Solid Edge part; units mm, degrees
sketch "Sketch1" plane through (0, 0, 0) normal (0, 0, 1) x (1, 0, 0)
  line L0 (-16, -30) -> (16, -30)
  line L1 (16, -30) -> (16, 30)
  line L2 (16, 30) -> (-16, 30)
  line L3 (-16, 30) -> (-16, -30)
  dimension "D1" = 16
  dimension "D2" = 16
extrude "Protrusion1" add sketch "Sketch1" along normal blind 73
sketch "Sketch2" plane through (0, 0, 73) normal (0, 0, 1) x (1, 0, 0)
  circle A0 centre (0, -20) radius 2.35
  circle A1 centre (0, -2) radius 2.35
extrude "Extrusionsausschnitt_1" cut sketch "Sketch2" against normal blind 36
chamfer "Fase_3" distance 0.7 angle 60 2 edges at (-2.35, -2, 73) (-2.35, -20, 73) measured on face at (-10.9867, -19.4, 73)
chamfer "Fase_6" distance 3 angle 45 4 edges at (-16, 0, 73) (-16, 0, 0) (16, 0, 73) (16, 0, 0)
chamfer "Fase_7" distance 3 angle 45 2 edges at (0, -30, 73) (0, -30, 0)
sketch "Sketch3" plane through (-16, 0, 36.5) normal (-1, 0, 0) x (0, -1, 0)
  circle A0 centre (-20, 25) radius 2.35
  circle A1 centre (-20, -25) radius 2.35
  circle A2 centre (10, 0) radius 2.35
  dimension "D1" = 20
extrude "Cutout1" cut sketch "Sketch3" against normal through all
chamfer "Fase_9" distance 0.7 angle 60 6 edges at (-16, 22.35, 61.5) (-16, -7.65, 36.5) (-16, 22.35, 11.5) (16, 20, 59.15) (16, 20, 9.15) (16, -10, 34.15) measured on face at (-16, 20.6, 58.1633) measured on face at (16, -20.6, 58.1633)
sketch "Sketch4" plane through (-16, 0, 36.5) normal (-1, 0, 0) x (0, -1, 0)
  line L0 (-6.5, 36.5) -> (-30, 36.5)
  line L1 (-30, 36.5) -> (-30, 36)
  line L2 (-30, 36) -> (-6.5, 36)
  line L3 (-6.5, 36) -> (-6.5, 36.5)
  line L4 (-30, -36.5) -> (-6.5, -36.5)
  line L5 (-6.5, -36.5) -> (-6.5, -36)
  line L6 (-6.5, -36) -> (-30, -36)
  line L7 (-30, -36) -> (-30, -36.5)
  dimension "D1" = 30
  dimension "D2" = 30
extrude "Cutout2" cut sketch "Sketch4" against normal through all
sketch "Sketch5" plane through (0, 30, 36.5) normal (0, 1, 0) x (1, 0, 0)
  line L0 (-16, 33.5) -> (-13.5, 36)
  line L1 (-13.5, 36) -> (13.5, 36)
  line L2 (13.5, 36) -> (16, 33.5)
  line L3 (16, 33.5) -> (16, -33.5)
  line L4 (16, -33.5) -> (13.5, -36)
  line L5 (13.5, -36) -> (-13.5, -36)
  line L6 (-13.5, -36) -> (-16, -33.5)
  line L7 (-16, -33.5) -> (-16, 33.5)
extrude "Extrusionsausprägung_2" add sketch "Sketch5" along normal blind 26
sketch "Sketch6" plane through (0, 36.25, 72.5) normal (0, 0, 1) x (0, 1, 0)
  circle A0 centre (9.75, 0) radius 2.35
  dimension "D1" = 9.75
extrude "Cutout3" cut sketch "Sketch6" against normal through all
chamfer "Fase_10" distance 0.7 angle 60 2 edges at (0, 43.65, 72.5) (-2.35, 46, 0.5) measured on face at (8.73, 48.245, 72.5) measured on face at (8.73, 14.255, 0.5)
sketch "Sketch7" plane through (0, 56, 36.5) normal (0, 1, 0) x (-1, 0, 0)
  line L0 (-13.5, 36) -> (-16, 33.5)
  line L1 (-16, 33.5) -> (-16, -33.5)
  line L2 (-16, -33.5) -> (-13.5, -36)
  line L3 (-13.5, -36) -> (13.5, -36)
  line L4 (13.5, -36) -> (16, -33.5)
  line L5 (16, -33.5) -> (16, 33.5)
  line L6 (16, 33.5) -> (13.5, 36)
  line L7 (13.5, 36) -> (-13.5, 36)
extrude "Extrusionsausprägung_3" add sketch "Sketch7" along normal blind 4
properties material "Nylon, allgemein"
Check sheet for the modelled part. Datum: model origin and axes. Units: mm. A direction names the side the tool comes from. Round coordinates to 2 decimals unless told otherwise and drop trailing zeros. Loops run counter-clockwise (first coordinate to the right, second up) from the corner with the lowest first, then second, coordinate; pieces in that order, holes last. Notation, with made-up numbers: (65.25, 88.5) -> (112.25, 88.5) arc R12 ccw to (112.25, 111.5) -> close; hole circle Ø1 at (59.25, 73.5). An arc over 180 degrees is marked (long way). Write item = value, one per line. Start each with the question number.
1) Sectioned sample at C-C, the plane y = -10. Record the cut outline in (x, z).
2) Sectioned sample at A-A, the plane x = 0. State how many separate pieces and enclosed holes the cut face has, plus the area to 3 significant figures.
3) Release check for a two-part mould opening along X. For faces 1 (the cylindrical face through (-0.509, -22.294, 54.637)), 2 (the flat face through (0, -28, 1)), 3 (the flat face through (-14, 14, 1)) record: released by +X, released by -X, zero draft, split by the parting line, or undercut.
4) Set-up check for faces 4 (the flat face through (0, 33, 0.5)), 5 (the flat face through (0, -10, 73)): record each of +Z, -Z, +X, -X, +Y, -Y from which the full face is reachable in a straight line by a thin tool's end or side.
5) Sectioned sample at B-B, the plane y = 20. Record the cut outline in (x, z), plus the area to 3 significant figures.
6) Sectioned sample at D-D, the plane z = 41.5. Record the cut outline in (x, y).
7) Gauge pin test, flat ends, axial feed: pin 1 Ø4 at (y, z) = (20, 11.5) entering from -X; pin 2 Ø8 at (x, y) = (-5, 40.5) entering from +Z; pin 3 Ø3 at (x, y) = (0, -20) entering from +Z; pin 4 Ø6 at (x, y) = (0, -2) entering from +Z. Record the tip position at first contact, or that the pin passes through.
8) Thickness scan on probe 1 along Y at (x, z) = (0, 56.5); probe 2 along X at (y, z) = (46, 47); probe 3 along Y at (x, z) = (1, 36). Record the ranges inside material, lowest first.
Results are:
q1.outline = (-16, 3) -> (-13, 0) -> (13, 0) -> (16, 3) -> (16, 33.45) -> (14.79, 34.15) -> (-14.79, 34.15) -> (-16, 33.45) -> close; (-16, 39.55) -> (-14.79, 38.85) -> (14.79, 38.85) -> (16, 39.55) -> (16, 70) -> (13, 73) -> (-13, 73) -> (-16, 70) -> close
q2.separate_pieces = 2
q2.enclosed_holes = 3
q2.area = 5,780 mm^2
q3.face_1 = undercut
q3.face_2 = zero draft
q3.face_3 = released by -X
q4.face_4 = -Z, +X, -X, +Y
q4.face_5 = +Z, +X, -X, +Y, -Y
q5.outline = (-16, 3) -> (-13.5, 0.5) -> (13.5, 0.5) -> (16, 3) -> (16, 8.45) -> (14.79, 9.15) -> (-14.79, 9.15) -> (-16, 8.45) -> close; (-16, 14.55) -> (-14.79, 13.85) -> (14.79, 13.85) -> (16, 14.55) -> (16, 58.45) -> (14.79, 59.15) -> (-14.79, 59.15) -> (-16, 58.45) -> close; (-16, 64.55) -> (-14.79, 63.85) -> (14.79, 63.85) -> (16, 64.55) -> (16, 70) -> (13.5, 72.5) -> (-13.5, 72.5) -> (-16, 70) -> close
q5.area = 1,990 mm^2
q6.outline = (-16, -30) -> (16, -30) -> (16, 60) -> (-16, 60) -> close; hole circle Ø4.7 at (0, -20); hole circle Ø4.7 at (0, -2); hole circle Ø4.7 at (0, 46)
q7.pin_1 = through
q7.pin_2 = 72.5
q7.pin_3 = 37
q7.pin_4 = 72.91
q8.probe_1 = -30 to -22.35, -17.65 to -4.35, 0.35 to 43.65, 48.35 to 60
q8.probe_2 = -16 to -2.35, 2.35 to 16
q8.probe_3 = -30 to -12.3, -7.7 to 43.87, 48.13 to 60
